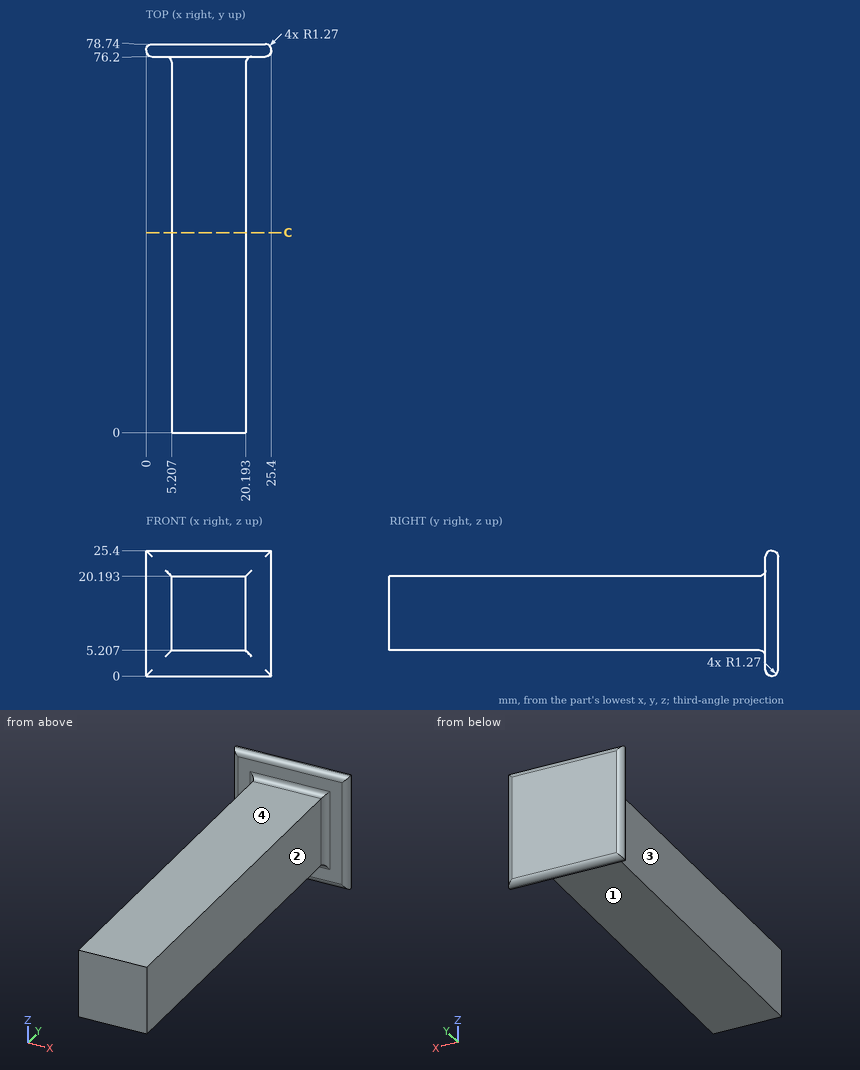
Input: dimensioned drawing with shaded views. Units: mm. Origin: part minimum x, y, z. A direction names the side the tool comes from. Round coordinates to 2 decimals unless told otherwise and drop trailing zeros. Write each loop counter-clockwise with the first axis right and the second up, starting at its lowest first coordinate (ties: lowest second). Pieces come first, ordered by that corner, then holes. Notation, with made-up numbers: (-12, 47.25) -> (21, 47.25) arc R20 cw to (21, 68.25) -> close; hole circle Ø11 at (33.5, -27). An arc over 180 degrees is marked (long way). Use CSV: the item, a comma, the result in double quotes. Start each with the question number.
Q1. Line query: L1, parallel to Z at x = 18.5, y = 38; L2, parallel to Y at x = 14.25, z = 22.75. Output: solid intervals per line, ascending.
Q2. First-contact query: pin 1 Ø4 at (y, z) = (57.5, 20) entering from +X; pin 2 Ø12 at (x, y) = (12, 41.5) entering from -Z; pin 3 Ø7.5 at (x, y) = (13, 36) entering from +Z. Flat tips, straight axial feed; report the tip coordinate or a pass-through.
Q3. Reachability of the marked faces 1, 2, 3 and 4 from +Z, -Z, +X, -X, +Y, -Y: full face, straight path, thin tool, end or side. Return the list, or none.
Q4. Section C-C (y = 40.5). Return loops of the section in (x, z).
Result sheet:
1,L1,"5.21 to 20.19"
1,L2,"76.2 to 78.74"
2,pin 1,"x = 20.19"
2,pin 2,"z = 5.21"
2,pin 3,"z = 20.19"
3,face 1,"-Z, +X, -X, -Y"
3,face 2,"+Z, -Z, +X, -Y"
3,face 3,"+Z, -Z, -X, -Y"
3,face 4,"+Z, +X, -X, -Y"
4,outline,"(5.21, 5.21) -> (20.19, 5.21) -> (20.19, 20.19) -> (5.21, 20.19) -> close"
